```python
from build123d import *

# Parameters (mm, degrees)
SKETCH1_W           = 238
SKETCH1_H           = 13
BOSS_EXTRUDE1_DEPTH = 3
SKETCH2_W           = 238
SKETCH2_H           = 3
BOSS_EXTRUDE2_DEPTH = 24
SKETCH3_W           = 14
SKETCH3_H           = 26
BOSS_EXTRUDE3_DEPTH = 3
SKETCH5_W           = 14
SKETCH5_H           = 23
BOSS_EXTRUDE5_DEPTH = 3


with BuildPart() as part:
    # Sketch1 → Boss-Extrude1 (new body)
    with BuildSketch(Plane(origin=(0, 0, 0), x_dir=(1, 0, 0), z_dir=(0, 1, 0))):
        with Locations((-119, -6.5)):
            Rectangle(SKETCH1_W, SKETCH1_H)
    extrude(amount=BOSS_EXTRUDE1_DEPTH)

    # Sketch2 → Boss-Extrude2 (add)
    with BuildSketch(Plane(origin=(0, 3, 0), x_dir=(1, 0, 0), z_dir=(0, 1, 0))):
        with Locations((-119, -1.5)):
            Rectangle(SKETCH2_W, SKETCH2_H)
    extrude(amount=BOSS_EXTRUDE2_DEPTH)

    # Sketch3 → Boss-Extrude3 (add)
    with BuildSketch(Plane.XZ):
        with Locations((-7, 13)):
            Rectangle(SKETCH3_W, SKETCH3_H)
    extrude(amount=-BOSS_EXTRUDE3_DEPTH)

    # Sketch5 → Boss-Extrude5 (add)
    with BuildSketch(Plane(origin=(0, 3, 0), x_dir=(1, 0, 0), z_dir=(0, 1, 0))):
        with Locations((-231, -14.5)):
            Rectangle(SKETCH5_W, SKETCH5_H)
    extrude(amount=-BOSS_EXTRUDE5_DEPTH)


solid = part.part
```
Check sheet for the modelled part. Datum: model origin and axes. Units: mm. A direction names the side the tool comes from. Give positions to 0.01 mm unless a question says otherwise; leave off trailing zeros. Order: outer loops, then holes, each group sorted by start corner. A loop starts at its lowest first (then second) coordinate and runs counter-clockwise, first axis right, second up. Notation, with made-up numbers: (22.25, 5.5) -> (31.25, 5.5) arc R13 cw to (31.25, 28.5) -> close; hole circle Ø8 at (-19.75, -27). An arc over 180 degrees is marked (long way). Return JSON: item names as keys, results as strings.
1. Set-up check for faces 1 (the flat face through (-121, 15, 3)), 2 (the flat face through (0, 8, 2)): record each of +Z, -Z, +X, -X, +Y, -Y from which the full face is reachable in a straight line by a thin tool's end or side.
From the geometry:
{"face 1": "+Z, +X, -X, +Y", "face 2": "+Z, -Z, +X, +Y, -Y"}
2. Go/stop test with flat-tipped pins: P1, Ø3.5, axis at x = -168, y = 1.5, coming from the +Z side; P2, Ø1.5, axis at x = -68, y = 5, coming from the +Z side. Record where each tip stops, or that it passes through.
From the geometry:
{"P1": "z = 13", "P2": "z = 3"}
3. Material ranges on probe 1 along X at (y, z) = (2.5, 17.75); probe 2 along Z at (x, y) = (-43.5, 5.25), recorded low to high. Write a range as [from, to].
From the geometry:
{"probe 1": "[-238, -224], [-14, 0]", "probe 2": "[0, 3]"}
4. Cross-section at C-C, the plane y = 8. Record the cut outline in (x, z), plus the area to 3 significant figures.
From the geometry:
{"outline": "(-238, 0) -> (0, 0) -> (0, 3) -> (-238, 3) -> close", "area": "714 mm^2"}
5. Cross-section at B-B, the plane x = -36.5. Record the cut outline in (y, z), plus the area to 3 significant figures.
From the geometry:
{"outline": "(0, 0) -> (27, 0) -> (27, 3) -> (3, 3) -> (3, 13) -> (0, 13) -> close", "area": "111 mm^2"}
6. Cross-section at A-A, the plane z = 16. Record the cut outline in (x, y).
From the geometry:
{"outline": "(-238, 0) -> (-224, 0) -> (-224, 3) -> (-238, 3) -> close; (-14, 0) -> (0, 0) -> (0, 3) -> (-14, 3) -> close"}
